Check sheet for the modelled part. Datum: model origin and axes. Units: mm. A direction names the side the tool comes from. Give positions to 0.01 mm unless a question says otherwise; leave off trailing zeros. Order: outer loops, then holes, each group sorted by start corner. A loop starts at its lowest first (then second) coordinate and runs counter-clockwise, first axis right, second up.
```python
from build123d import *

# Parameters (mm, degrees)
PAD_DEPTH = 2


with BuildPart() as part:
    # Sketch → Pad (new body)
    with BuildSketch(Plane.XY):
        with BuildLine():
            Line((-60.105615, 45.533643), (-54.466598, 48.091796))
            ThreePointArc((-52.403313, 47.678624), (-53.368379, 48.217678), (-54.466598, 48.091796))
            Line((-52.403313, 47.678624), (-51.737988, 46.96393))
            ThreePointArc((-51.737988, 46.96393), (-50.585163, 46.283393), (-49.247664, 46.340273))
            Line((-49.247664, 46.340273), (-46.846974, 47.163608))
            ThreePointArc((-44.679417, 47.414663), (-45.776747, 47.406135), (-46.846974, 47.163608))
            Line((-44.679417, 47.414663), (-39.67485, 46.913708))
            Line((-39.67485, 46.913708), (-39.952934, 45.634525))
            Line((-39.952934, 45.634525), (-44.774068, 46.226029))
            ThreePointArc((-44.774068, 46.226029), (-45.579656, 46.243017), (-46.372273, 46.098043))
            Line((-46.372273, 46.098043), (-50.39025, 44.934378))
            ThreePointArc((-52.180316, 45.54252), (-51.380911, 44.956967), (-50.39025, 44.934378))
            Line((-52.180316, 45.54252), (-52.510514, 45.991705))
            ThreePointArc((-52.510514, 45.991705), (-53.67937, 46.769354), (-55.074387, 46.611594))
            Line((-55.074387, 46.611594), (-60.105615, 44.103531))
            Line((-60.105615, 44.103531), (-60.105615, 45.533643))
        make_face()
    extrude(amount=PAD_DEPTH)


solid = part.part
```
Q1. Material ranges on line 1 (X direction, y = 47.5, z = 0.85); line 2 (Y direction, x = -56, z = 1.9); line 3 (Y direction, x = -47, z = 1.7), recorded low to high.
Q2. Sectioned sample at D-D, the plane y = 47.9. Record the cut outline in (x, z).
Q3. Tool access check on faces 1 (the flat face through (-39.812, 46.283, 0.986)), 2 (the flat face through (-57.555, 45.375, 0.986)), 3 (the flat face through (-48.064, 46.746, 0.986)). Record the directions out of +Z, -Z, +X, -X, +Y, -Y that give a thin tool (end or side, any length) a straight path to the whole face; none if there is none.
Q4. Sectioned sample at C-C, the plane x = -41.5. Record the cut outline in (y, z), plus the area to 3 significant figures.
Q5. Sectioned sample at B-B, the plane y = 45.35. Record the cut outline in (x, z), plus the area to 3 significant figures.
Q6. Sectioned sample at A-A, the plane z = 1.7. Record the cut outline in (x, y), plus the area to 3 significant figures.
Filled in:
1. line 1: x = -55.77 to -52.24
1. line 2: y = 46.15 to 47.4
1. line 3: y = 45.92 to 47.11
2. outline: (-54.89, 0) - (-52.65, 0) - (-52.65, 2) - (-54.89, 2) - close
3. face 1: +Z, -Z, +X, -Y
3. face 2: +Z, -Z, -Y
3. face 3: +Z, -Z, +Y
4. outline: (45.82, 0) - (47.1, 0) - (47.1, 2) - (45.82, 2) - close
4. area: 2.54 mm2
5. outline: (-60.11, 0) - (-57.61, 0) - (-57.61, 2) - (-60.11, 2) - close; (-52.01, 0) - (-48.96, 0) - (-48.96, 2) - (-52.01, 2) - close
5. area: 11.1 mm2
6. outline: (-60.11, 44.1) - (-55.07, 46.61) arc R2.05 cw to (-52.51, 45.99) - (-52.18, 45.54) arc R1.65 ccw to (-50.39, 44.93) - (-46.37, 46.1) arc R4 cw to (-44.77, 46.23) - (-39.95, 45.63) - (-39.67, 46.91) - (-44.68, 47.41) arc R5.11 ccw to (-46.85, 47.16) - (-49.25, 46.34) arc R2.36 cw to (-51.74, 46.96) - (-52.4, 47.68) arc R1.8 ccw to (-54.47, 48.09) - (-60.11, 45.53) - close
6. area: 26.7 mm2
